The model under review builds one solid part; all positions refer to its coordinate system, in mm. A direction names the side the tool comes from. Round coordinates to 2 decimals unless told otherwise and drop trailing zeros. Order: outer loops, then holes, each group sorted by start corner. A loop starts at its lowest first (then second) coordinate and runs counter-clockwise, first axis right, second up. Notation, with made-up numbers: (59, 4.5) -> (74, 4.5) arc R21 cw to (74, 21.5) -> close; hole circle Ø2 at (79.25, 29.25). An arc over 180 degrees is marked (long way). Use a Markdown table: item, result. Add a question column.
Autodesk Inventor part; units mm, degrees
ref_plane "YZ Plane" through (0, 0, 0) normal (1, 0, 0) x (0, 1, 0)
ref_plane "XZ Plane" through (0, 0, 0) normal (0, 1, 0) x (-1, 0, 0)
ref_plane "XY Plane" through (0, 0, 0) normal (0, 0, 1) x (1, 0, 0)
sketch "Szkic1" plane through (0, 0, 0) normal (0, 1, 0) x (-1, 0, 0)
  line L0 (-19, 622) -> (11, 622) construction
  line L1 (11, 622) -> (147, 486) construction
  line L2 (147, 486) -> (176.8016, 486) construction
  line L3 (176.8016, 486) -> (176.8016, 461) construction
  line L4 (-19, 622) -> (-19, 609.2855) construction
  line L5 (-19, 609.2855) -> (176.8016, 413.4839) construction
  line L6 (176.8016, 413.4839) -> (176.8016, 461) construction
  line L7 (176.8016, 486) -> (176.8016, 1189) construction
  line L8 (146.8016, 1189) -> (146.8016, 533) construction
  line L9 (246.8016, 495.9837) -> (246.8016, 1189) construction
  line L10 (-47, 922) -> (309, 922) construction
  line L11 (-42, 1147) -> (293, 1147) construction
  line L12 (12.455, 587.5586) -> (52.6586, 1162.4969)
  line L13 (67.6221, 1176.4505) -> (79.6466, 1176.4505)
  line L14 (147, 486) -> (147, 443.2855) construction
  line L15 (147, 486) -> (142.6159, 490.3841) construction
  line L16 (142.6159, 490.3841) -> (121.2587, 469.0268) construction
  line L17 (18.2642, 572.0213) -> (139.5006, 450.7849)
  line L18 (-99.7145, 690) -> (195.2855, 395) construction
  line L19 (172.3089, 417.9767) -> (172.3089, 447.856) construction
  line L20 (176.8016, 486) -> (315.5485, 347.2531) construction
  line L21 (141.5331, 491.4664) -> (138.3972, 536.3123)
  line L22 (162.3089, 477.5127) -> (156.4966, 477.5127)
  line L23 (162.3089, 447.856) -> (146.5717, 447.856)
  arc A0 (12.455, 587.5586) -> (18.2642, 572.0213) centre (32.4063, 586.1635) ccw
  line L24 (142.4296, 447.856) -> (172.3089, 417.9767) construction
  line L25 (172.3089, 457.856) -> (172.3089, 467.5127)
  arc A1 (141.5331, 491.4664) -> (156.4966, 477.5127) centre (156.4966, 492.5127) ccw
  arc A2 (172.3089, 467.5127) -> (162.3089, 477.5127) centre (162.3089, 467.5127) ccw
  arc A3 (162.3089, 447.856) -> (172.3089, 457.856) centre (162.3089, 457.856) ccw
  arc A4 (139.5006, 450.7849) -> (146.5717, 447.856) centre (146.5717, 457.856) ccw
  arc A5 (94.6101, 1162.4969) -> (79.6466, 1176.4505) centre (79.6466, 1161.4505) ccw
  arc A6 (67.6221, 1176.4505) -> (52.6586, 1162.4969) centre (67.6221, 1161.4505) ccw
  line L26 (141.5331, 491.4664) -> (144.7446, 445.541) construction
  line L27 (141.5331, 491.4664) -> (141.5331, 448.7524) construction
  line L28 (-28.6025, 640.2452) -> (163.5033, 448.1395) construction
  line L29 (47.7855, 542.5) -> (47.7855, 585.2145) construction
  line L30 (-4, 664.8499) -> (-4, 551.9978) construction
  line L31 (11, 622) -> (11, 579.2855) construction
  line L32 (11, 579.2855) -> (15.3841, 574.9015) construction
  line L33 (15.3841, 574.9015) -> (36.7413, 596.2587) construction
  line L34 (161.8016, 495.9837) -> (161.8016, 402) construction
  line L35 (104.2165, 1025.1187) -> (100.7287, 1074.9969) construction
  line L36 (100.7287, 1074.9969) -> (125.6678, 1076.7408)
  line L37 (125.6678, 1076.7408) -> (129.1556, 1026.8626)
  line L38 (129.1556, 1026.8626) -> (104.2165, 1025.1187)
  line L39 (100.7287, 1074.9969) -> (97.9384, 1114.8994)
  line L40 (104.2165, 1025.1187) -> (100.7287, 1074.9969) construction
  line L41 (73.1142, 1047.0024) -> (72.9747, 1048.9975)
  line L42 (74.8303, 1051.1322) -> (91.7889, 1052.318)
  line L43 (93.9236, 1050.4624) -> (94.0631, 1048.4673)
  line L44 (92.2075, 1046.3326) -> (75.2489, 1045.1468)
  line L45 (93.9933, 1049.4649) -> (102.4726, 1050.0578) construction
  line L46 (102.4726, 1050.0578) -> (114.4434, 1050.8949) construction
  arc A7 (74.8303, 1051.1322) -> (72.9747, 1048.9975) centre (74.9699, 1049.137) ccw
  arc A8 (73.1142, 1047.0024) -> (75.2489, 1045.1468) centre (75.1094, 1047.1419) ccw
  arc A9 (93.9236, 1050.4624) -> (91.7889, 1052.318) centre (91.9284, 1050.3229) ccw
  arc A10 (92.2075, 1046.3326) -> (94.0631, 1048.4673) centre (92.068, 1048.3278) ccw
  line L47 (116.505, 1021.4131) -> (111.1905, 1097.4131) construction
  line L48 (114.9666, 1043.4131) -> (113.9202, 1058.3766) construction
  line L49 (118.2139, 1047.1488) -> (117.6558, 1055.1293)
  line L50 (110.6729, 1054.641) -> (111.2309, 1046.6605)
  arc A11 (111.2309, 1046.6605) -> (118.2139, 1047.1488) centre (114.7224, 1046.9046) ccw
  arc A12 (117.6558, 1055.1293) -> (110.6729, 1054.641) centre (114.1644, 1054.8851) ccw
  line L51 (47.9957, 591.7873) -> (80.3202, 559.4628)
  line L52 (105.8902, 571.1158) -> (83.3114, 894.0086)
  line L53 (75.3309, 901.4505) -> (71.9379, 901.4505)
  line L54 (63.9574, 894.0086) -> (43.6388, 603.4402)
  arc A13 (43.6388, 603.4402) -> (47.9957, 591.7873) centre (58.6023, 602.3939) ccw
  arc A14 (80.3202, 559.4628) -> (105.8902, 571.1158) centre (90.9268, 570.0694) ccw
  arc A15 (83.3114, 894.0086) -> (75.3309, 901.4505) centre (75.3309, 893.4505) ccw
  arc A16 (71.9379, 901.4505) -> (63.9574, 894.0086) centre (71.9379, 893.4505) ccw
  line L55 (97.9384, 1114.8994) -> (96.8921, 1129.8629) construction
  line L56 (96.8921, 1129.8629) -> (101.8799, 1130.2117)
  line L57 (101.8799, 1130.2117) -> (102.9263, 1115.2482)
  line L58 (102.9263, 1115.2482) -> (97.9384, 1114.8994)
  line L59 (97.9384, 1114.8994) -> (112.9384, 1114.8994) construction
  line L60 (97.9384, 1114.8994) -> (96.8921, 1129.8629) construction
  line L61 (96.8921, 1129.8629) -> (94.6101, 1162.4969)
  line L62 (107.0068, 985.2161) -> (111.9946, 985.5649)
  line L63 (111.9946, 985.5649) -> (113.041, 970.6014)
  line L64 (113.041, 970.6014) -> (108.0531, 970.2527)
  line L65 (107.0068, 985.2161) -> (104.2165, 1025.1187)
  line L66 (108.0531, 970.2527) -> (107.0068, 985.2161) construction
  line L67 (138.3972, 536.3123) -> (137.3509, 551.2758)
  line L68 (137.3509, 551.2758) -> (143.3362, 551.6943)
  line L69 (143.3362, 551.6943) -> (144.3826, 536.7308)
  line L70 (144.3826, 536.7308) -> (138.3972, 536.3123)
  line L71 (138.3972, 536.3123) -> (153.3972, 536.3123) construction
  line L72 (131.9463, 1052.1188) -> (62.9796, 1047.2962) construction
  line L73 (137.3509, 551.2758) -> (108.0531, 970.2527)
  line L74 (138.3972, 536.3123) -> (137.3509, 551.2758) construction
  line L75 (138.4533, 621.5238) -> (139.4996, 606.5603)
  line L76 (139.4996, 606.5603) -> (133.5142, 606.1418)
  line L77 (132.4679, 621.1052) -> (138.4533, 621.5238)
  line L78 (133.5142, 606.1418) -> (132.4679, 621.1052)
  line L79 (133.5703, 691.3533) -> (134.6167, 676.3898)
  line L80 (134.6167, 676.3898) -> (128.6313, 675.9713)
  line L81 (127.5849, 690.9347) -> (133.5703, 691.3533)
  line L82 (128.6313, 675.9713) -> (127.5849, 690.9347)
  line L83 (128.6874, 761.1827) -> (129.7337, 746.2193)
  line L84 (129.7337, 746.2193) -> (123.7483, 745.8007)
  line L85 (122.702, 760.7642) -> (128.6874, 761.1827)
  line L86 (123.7483, 745.8007) -> (122.702, 760.7642)
  line L87 (123.8044, 831.0122) -> (124.8508, 816.0488)
  line L88 (124.8508, 816.0488) -> (118.8654, 815.6302)
  line L89 (117.819, 830.5937) -> (123.8044, 831.0122)
  line L90 (118.8654, 815.6302) -> (117.819, 830.5937)
  line L91 (118.9215, 900.8417) -> (119.9678, 885.8783)
  line L92 (119.9678, 885.8783) -> (113.9824, 885.4597)
  line L93 (112.9361, 900.4232) -> (118.9215, 900.8417)
  line L94 (113.9824, 885.4597) -> (112.9361, 900.4232)
  point P0 (0, 0)
  point P1 (11.8192, 578.4663)
  point P2 (53.6344, 1176.4505)
  point P3 (93.6344, 1176.4505)
  point P4 (172.3089, 477.5127)
  point P5 (142.5089, 477.5127)
  point P6 (47.7855, 563.8572)
  point P7 (27.4914, 584.1513)
  point P8 (148.7868, 462.856)
  point P9 (158.9877, 462.856)
  point P10 (93.2396, 518.4032)
  point P11 (60.3655, 551.2773)
  point P12 (126.1136, 485.5291)
  point P13 (72.8352, 1050.9927)
  point P14 (93.7841, 1052.4575)
  point P15 (118.4866, 1051.1776)
  dimension "d0" = 30
  dimension "d1" = 100
  dimension "d2" = 225
  dimension "d3" = 300
  dimension "d4" = 40
  dimension "d5" = 6.2
  dimension "d14" = 94
  dimension "d16" = 94
  dimension "d18" = 29.8
  dimension "d22" = 700.6445
  dimension "d23" = 20
  dimension "d24" = 15
  dimension "d25" = 10
  dimension "d26" = 10
  dimension "d28" = 15.7372
  dimension "d29" = 15
  dimension "d30" = 42.714
  dimension "d31" = 42.7145
  dimension "d32" = 21.3572
  dimension "d33" = 30
  dimension "d34" = 15
  dimension "d35" = 6.2
  dimension "d39" = 15.0364
  dimension "d40" = 15
  dimension "d43" = 23.5221
  dimension "d45" = 13.3212
  dimension "d46" = 15
  dimension "d47" = 131.4963
  dimension "d48" = 65.7481
  dimension "d49" = 32.8741
  dimension "d50" = 32.8741
  dimension "d51" = 50
  dimension "d52" = 25
  dimension "d53" = 87.5
  dimension "d56" = 21
  dimension "d57" = 8.5
  dimension "d58" = 12
  dimension "d60" = 2
  dimension "d62" = 6
  dimension "d63" = 15
  dimension "d64" = 7
  dimension "d65" = 25
  dimension "d66" = 275
  dimension "d67" = 30
  dimension "d68" = 30
  dimension "d69" = 35
  dimension "d70" = 15
  dimension "d71" = 8
  dimension "d72" = 15
  dimension "d73" = 94
  dimension "d74" = 5
  dimension "d75" = 40
  dimension "d78" = 145
  dimension "d83" = 15
  dimension "d84" = 94
  dimension "d85" = 6
  dimension "d86" = 3
  dimension "d87" = 16.014
  dimension "d88" = 25
  dimension "d99" = 70
  dimension "d113" = 420
extrude "Wyciągnięcie proste1" add sketch "Szkic1" along normal blind 5
hole "Otwór1" at (-27.4914, 0, 584.1513) at (-148.7868, 0, 462.856) at (-158.9877, 0, 462.856) at (-93.2396, 0, 518.4032) at (-60.3655, 0, 551.2773) at (-126.1136, 0, 485.5291) direction (0, 1, 0) diameter 4.5 depth 8 tip angle 118
equation "\"d16\" = d14"
properties part number "nowy_bok"
Q1. Mouldability with a two-part tool opening along X and no side actions: class faces 1 (the cylindrical face through (-97.38, 2.46, 556.53)), 2 (the flat face through (-91, 0, 817)), 3 (the flat face through (-78.034, 2.465, 512.252)) as pulls with the +X half, pulls with the -X half, needs draft (parallel to the pull), parting line crosses it, or undercut.
Q2. Insertion check: pin 1 (4 mm diameter, centred on x = -27.49, z = 584.15, fed in from +Y); pin 2 (2.5 mm diameter, centred on x = -159.5, y = 2.5, fed in from +Z); pin 3 (3 mm diameter, centred on y = 2.5, z = 594.5, fed in from +X); pin 4 (1.5 mm diameter, centred on y = 0.5, z = 924.5, fed in from +X). Each pin has a flat end and moves straight along its axis. Give the tip position at first contact, or say it passes through.
Q3. Machinability: for faces 4 (the flat face through (-53.94, 2.46, 750.76)), 5 (the cylindrical face through (-146.38, 2.46, 481.44)), 6 (the cylindrical face through (-89.76, 2.46, 1172.53)), which of the approach directions +Z, -Z, +X, -X, +Y, -Y give a long, thin tool a straight path to every point of the face, cutting with its end or side? Answer none if there is none.
Q4. Add section A-A (z = 871.5). Write out the cut boundary in (x, y).
Q5. Wall thickness on line 1 (X direction, y = 0.45, z = 1044); line 2 (X direction, y = 0.3, z = 793); line 3 (Z direction, x = -66.5, y = 3.8): over which ranges is each line inside the solid? List them lowest first. Write a range as [from, to].
Q6. Add section B-B (y = 3.8). State how many separate pieces and enclosed holes the cut face has, then the cut area to 3 significant figures.
Report:
| question | item | result |
|---|---|---|
| 1 | face 1 | undercut |
| 1 | face 2 | needs draft |
| 1 | face 3 | pulls with the +X half |
| 2 | pin 1 | passes through |
| 2 | pin 2 | stops at z = 477.51 |
| 2 | pin 3 | stops at x = -12.84 |
| 2 | pin 4 | stops at x = -35.96 |
| 3 | face 4 | +Y, -Y |
| 3 | face 5 | -X, +Y, -Y |
| 3 | face 6 | +Z, -X, +Y, -Y |
| 4 | outline | (-114.96, 0) -> (-84.89, 0) -> (-84.89, 5) -> (-114.96, 5) -> close; (-62.38, 0) -> (-32.31, 0) -> (-32.31, 5) -> (-62.38, 5) -> close |
| 5 | line 1 | x = [-127.96, -116.68], [-112.77, -44.37] |
| 5 | line 2 | x = [-120.45, -90.37], [-56.89, -26.82] |
| 5 | line 3 | z = [523.79, 573.28], [899.32, 1176.41] |
| 6 | separate pieces | 1 |
| 6 | enclosed holes | 9 |
| 6 | area | 45,800 mm² |
